from build123d import *

# Parameters (mm, degrees)
BOSS_EXTRUDE1_DEPTH = 38
SKETCH2_W           = 22
SKETCH2_H           = 10
CUT_EXTRUDE1_DEPTH  = 76.040117824
SKETCH3_W           = 14
SKETCH3_H           = 10


with BuildPart() as part:
    # Sketch1 → Boss-Extrude1 (new body)
    with BuildSketch(Plane.XY):
        Polygon((4.047792592, 41.073340295), (-3.952207408, 41.073340295), (-3.952207408, 22.406673629), (-17.952207408, 22.406673629), (-17.952207408, 14.406673629), (46.047792592, 14.406673629), (46.047792592, 22.406673629), (32.047792592, 22.406673629), (32.047792592, 41.073340295), (24.047792592, 41.073340295), (24.047792592, 25.700791276), (4.047792592, 25.700791276), align=None)
    extrude(amount=BOSS_EXTRUDE1_DEPTH)

    # Sketch2 → Cut-Extrude1 (cut, through all)
    with BuildSketch(Plane(origin=(32.047792592, 0, 0), x_dir=(0, 0, -1), z_dir=(1, 0, 0))):
        with Locations((-19, 41.073340295)):
            Rectangle(SKETCH2_W, SKETCH2_H)
    extrude(amount=-CUT_EXTRUDE1_DEPTH, mode=Mode.SUBTRACT)

    # Sketch3 → Cut-Revolve1 (revolve, cut)
    with BuildSketch(Plane(origin=(46.047792592, 0, 0), x_dir=(0, 0, -1), z_dir=(1, 0, 0))):
        with Locations((-19, 14.406673629)):
            Rectangle(SKETCH3_W, SKETCH3_H)
    revolve(axis=Axis((46.047792592, 19.406673629, 12), (0, 0, 1)), mode=Mode.SUBTRACT)


solid = part.part
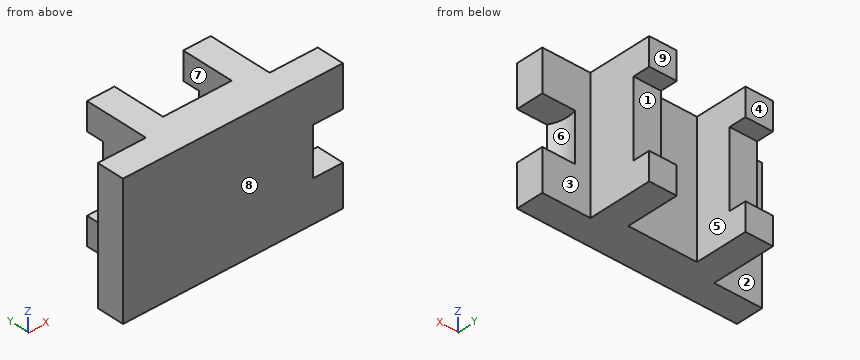
Build history of the part. All positions in model axes, mm. Face numbers are marked on the shaded views. A direction names the side the tool comes from. Give positions to 0.01 mm unless a question says otherwise; leave off trailing zeros. Write each loop counter-clockwise with the first axis right and the second up, starting at its lowest first coordinate (ties: lowest second). Pieces come first, ordered by that corner, then holes. Notation, with made-up numbers: (23, 32.5) - (31, 32.5) arc R21 cw to (31, 41.5) - close; hole circle Ø6 at (-23.5, 48.5). An arc over 180 degrees is marked (long way). Use one line per item in the form item = value. Start each with the question number.
1. Probe line 1 (X direction, y = 36, z = 14.5); line 2 (Z direction, x = 39.5, y = 18.5); line 3 (Z direction, x = 0, y = 36.5). List the from-to ranges inside material, lowest first. Write a range as [from, to].
2. Band-saw the part on B-B on x = 42. Write the cut outline in (y, z).
3. Drop flat-ended pins along their axis: pin 1 Ø1.5 at (y, z) = (25.5, 8.5) entering from +X; pin 2 Ø4.5 at (y, z) = (31, 10.5) entering from -X; pin 3 Ø4 at (x, z) = (0, 21.5) entering from +Y; pin 4 Ø8 at (x, y) = (-8, 36) entering from +Z. Give the stop position or say it passes through.
4. Band-saw the part on C-C on y = 38.5. Write the cut outline in (x, z), plus the area to 3 significant figures.
5. 3-axis set-ups, long thin cutter, end or side, ignore diameter. For the marked faces 1, 2, 3, 4 and 5: which of +Z, -Z, +X, -X, +Y, -Y reach the whole face in a straight line?
6. Band-saw the part on D-D on z = 27.5. Write the cut outline in (x, y), plus the area to 3 significant figures.
7. Two-plate mould, pull along Y, no slides. Class the marked faces 6, 7, 8 and 9: released by +Y, released by -Y, zero draft, split by the parting line, or undercut.
8. Band-saw the part on A-A on y = 33.5. Write the cut outline in (x, z), plus the area to 3 significant figures.
Conclusion:
q1.line_1 = [-3.95, 4.05], [24.05, 32.05]
q1.line_2 = [0, 12], [26, 38]
q1.line_3 = [0, 8], [30, 38]
q2.outline = (14.41, 0) - (22.41, 0) - (22.41, 12) - (14.41, 12) - close; (14.41, 26) - (22.41, 26) - (22.41, 38) - (14.41, 38) - close
q3.pin_1 = 32.05
q3.pin_2 = -3.95
q3.pin_3 = 36.07
q3.pin_4 = through
q4.outline = (-3.95, 0) - (4.05, 0) - (4.05, 8) - (-3.95, 8) - close; (-3.95, 30) - (4.05, 30) - (4.05, 38) - (-3.95, 38) - close; (24.05, 0) - (32.05, 0) - (32.05, 8) - (24.05, 8) - close; (24.05, 30) - (32.05, 30) - (32.05, 38) - (24.05, 38) - close
q4.area = 256 mm²
q5.face_1 = +X, -X, +Y
q5.face_2 = +Z, -Z, -X, +Y
q5.face_3 = +Z, -Z, +X, +Y
q5.face_4 = +Z, -Z, +X, -X, +Y
q5.face_5 = +Z, -Z, +Y
q6.outline = (-17.95, 14.41) - (46.05, 14.41) - (46.05, 22.41) - (32.05, 22.41) - (32.05, 36.07) - (24.05, 36.07) - (24.05, 25.7) - (4.05, 25.7) - (4.05, 36.07) - (-3.95, 36.07) - (-3.95, 22.41) - (-17.95, 22.41) - close
q6.area = 797 mm²
q7.face_6 = undercut
q7.face_7 = zero draft
q7.face_8 = released by -Y
q7.face_9 = released by +Y
q8.outline = (-3.95, 0) - (4.05, 0) - (4.05, 38) - (-3.95, 38) - close; (24.05, 0) - (32.05, 0) - (32.05, 38) - (24.05, 38) - close
q8.area = 608 mm²
